Work out the finished part from the listing and answer in its coordinate system (mm). A direction names the side the tool comes from. Round coordinates to 2 decimals unless told otherwise and drop trailing zeros. Order: outer loops, then holes, each group sorted by start corner. A loop starts at its lowest first (then second) coordinate and runs counter-clockwise, first axis right, second up. Notation, with made-up numbers: (32, 76) - (50, 76) arc R19 cw to (50, 98) - close; hole circle Ø8 at (-4.75, -22.5). An arc over 180 degrees is marked (long way). Use one line per item in the form item = value. Start each with the question number.
Q1. The part is cut by section A-A on z = 0. Determine the outline of the cut face in (x, y).
Q2. The part is cut by section C-C on y = 4. Determine the outline of the cut face in (x, z).
Q3. Given P1, Ø1, axis at x = 56, y = -1, coming from the -Z side; P2, Ø2, axis at x = 38, z = -1, coming from the +Y side; P3, Ø3, axis at x = 66.5, y = -3.5, coming from the +Z side, each flat-ended and moving along its own axis, determine where each tip first touches the part or whether it passes through.
Q4. Which of the six approach directions +Z, -Z, +X, -X, +Y, -Y give full straight-line access (tool end or side, diameter ignored) to faces 1 (the flat face through (105, 0, 2.5)), 2 (the flat face through (105, 0, -2.5)), 3 (the cylindrical face through (107.49, 0.54, 2.44)), 4 (the cylindrical face through (115, 3, 0))?
Q5. Find the intervals of material crossed by line 1 (Z direction, x = 67, y = 0); line 2 (X direction, y = -1.5, z = 4.25); line 3 (Y direction, x = 77, z = 2.5), in increasing order. Write a range as [from, to].
Q6. The part is cut by section B-B on x = 101. Determine the outline of the cut face in (y, z), plus the area to 3 significant figures.
Q7. The part is cut by section D-D on z = 5. Determine the outline of the cut face in (x, y), plus the area to 3 significant figures.
Q8. For a pull along X with two mould halves and no side action, classify faces 5 (the flat face through (19, -3, 1)), 6 (the flat face through (107, 2.7, -0.2)), 7 (the cylindrical face through (62, 3, 0)) as +X half, -X half, draft (parallel to the pull), parting line (faces both ways), or undercut.
from build123d import *

# Parameters (mm, degrees)
CHAMFER1_SIZE      = 0.5
SKETCH2_W          = 3.5
SKETCH2_H          = 12
CUT_EXTRUDE1_DEPTH = 4


with BuildPart() as part:
    # Sketch1 → Revolve1 (revolve)
    with BuildSketch(Plane.XY):
        Polygon((0, -6), (0, 0), (123, 0), (123, -3), (108.5, -3), (108, -2.5), (107, -2.5), (107, -3), (19, -3), (19, -6), align=None)
    revolve(axis=Axis((-26.391164048, 0, 0), (1, 0, 0)))

    # Chamfer1
    chamfer1_edges = [part.edges().sort_by_distance(p)[0] for p in [
        (123, 3, 0),
    ]]
    chamfer(chamfer1_edges, length=CHAMFER1_SIZE)

    # Sketch2 → Cut-Extrude1 (cut)
    with BuildSketch(Plane(origin=(107, 0, 0), x_dir=(0, 0, -1), z_dir=(1, 0, 0))):
        with Locations((-4.25, 0)):
            Rectangle(SKETCH2_W, SKETCH2_H)
    cut_extrude1 = extrude(amount=-CUT_EXTRUDE1_DEPTH, mode=Mode.SUBTRACT)

    # Mirror1: Cut-Extrude1 across plane
    add(cut_extrude1.mirror(Plane.XY), mode=Mode.SUBTRACT)


solid = part.part
Found:
q1.outline = (0, -6) - (19, -6) - (19, -3) - (107, -3) - (107, -2.5) - (108, -2.5) - (108.5, -3) - (122.5, -3) - (123, -2.5) - (123, 2.5) - (122.5, 3) - (108.5, 3) - (108, 2.5) - (107, 2.5) - (107, 3) - (19, 3) - (19, 6) - (0, 6) - close
q2.outline = (0, -4.47) - (19, -4.47) - (19, 4.47) - (0, 4.47) - close
q3.P1 = -2.96
q3.P2 = 3
q3.P3 = 2.24
q4.face_1 = +Z, +Y, -Y
q4.face_2 = -Z, +Y, -Y
q4.face_3 = none
q4.face_4 = +X
q5.line_1 = [-3, 3]
q5.line_2 = [0, 19]
q5.line_3 = [-1.66, 1.66]
q6.outline = circle Ø6 at (0, 0)
q6.area = 28.3 mm²
q7.outline = (0, -3.32) - (19, -3.32) - (19, 3.32) - (0, 3.32) - close
q7.area = 126 mm²
q8.face_5 = +X half
q8.face_6 = undercut
q8.face_7 = draft
